```python
from build123d import *

# Parameters (mm, degrees)
SKETCH1_R           = 12.5
SKETCH1_R_2         = 1.6
SKETCH1_R_3         = 1
BOSS_EXTRUDE1_DEPTH = 5
CUT_EXTRUDE1_DEPTH  = 6
CIRPATTERN1_COUNT   = 22


with BuildPart() as part:
    # Sketch1 → Boss-Extrude1 (new body)
    with BuildSketch(Plane.XY):
        Circle(SKETCH1_R)
        Circle(SKETCH1_R_2, mode=Mode.SUBTRACT)
        with Locations((2.5, -7.4)):
            Circle(SKETCH1_R_3, mode=Mode.SUBTRACT)
        with Locations((-2.5, -7.4)):
            Circle(SKETCH1_R_3, mode=Mode.SUBTRACT)
        with Locations((7.4, -2.5)):
            Circle(SKETCH1_R_3, mode=Mode.SUBTRACT)
        with Locations((-7.4, -2.694035424)):
            Circle(SKETCH1_R_3, mode=Mode.SUBTRACT)
        with Locations((-7.4, 2.5)):
            Circle(SKETCH1_R_3, mode=Mode.SUBTRACT)
        with Locations((-2.5, 7.4)):
            Circle(SKETCH1_R_3, mode=Mode.SUBTRACT)
        with Locations((2.5, 7.4)):
            Circle(SKETCH1_R_3, mode=Mode.SUBTRACT)
        with Locations((7.4, 2.5)):
            Circle(SKETCH1_R_3, mode=Mode.SUBTRACT)
    extrude(amount=BOSS_EXTRUDE1_DEPTH)

    # Sketch2 → Cut-Extrude1 (cut, through all)
    with BuildSketch(Plane.XY.offset(5)):
        Polygon((-9.204992805, 8.456837911), (-6.616673599, 6.940063806), (-5.995627184, 7.483135026), (-7.153657676, 10.250618608), (-7.456074993, 10.596457577), (-9.507410122, 8.80267688), align=None)
    cut_extrude1 = extrude(amount=-CUT_EXTRUDE1_DEPTH, mode=Mode.SUBTRACT)

    # CirPattern1: Cut-Extrude1 ×22 about axis
    cirpattern1_axis = Axis((0, 0, 0), (0, 0, 1))
    for i in range(1, CIRPATTERN1_COUNT):
        add(cut_extrude1.rotate(cirpattern1_axis, i * 360 / CIRPATTERN1_COUNT), mode=Mode.SUBTRACT)


solid = part.part
```
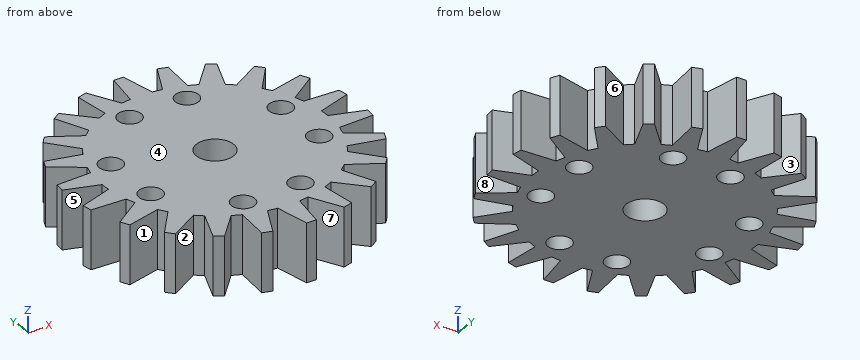
Here's how the part is built. I have some questions about the finished solid (model axes, mm). Face numbers are marked on the shaded views. A direction names the side the tool comes from. Give positions to 0.01 mm unless a question says otherwise; leave off trailing zeros. Write each loop counter-clockwise with the first axis right and the second up, starting at its lowest first coordinate (ties: lowest second). Pieces come first, ordered by that corner, then holes. Notation, with made-up numbers: M 85.25,40.25 L 120.25,40.25 A26 ccw 120.25,73.25 Z; hole C 15.25,-30 d2. An arc over 180 degrees is marked long. Put each result on its own line as item: value. Start each with the question number.
Item 1: Will this pin go through, and if not, where does the flat tip stop? pin 1 (2 mm diameter, centred on x = -7, z = 3, fed in from +Y).
Item 2: If we section it at D-D, the plane x = 2.5: Write out the boundary of the cut face in (y, z), then the cut area to 3 significant figures.
Item 3: I need wall thicknesses on L1, parallel to Y at x = 7.4, z = 1.85; L2, parallel to Y at x = 8.5, z = 0.35; L3, parallel to Y at x = 11.25, z = 2.45. Which ranges of each line are inside material? Lowest first, please. Write a range as from..to.
Item 4: If we section it at B-B, the plane x = 0: Write out the boundary of the cut face in (y, z), then the cut area to 3 significant figures.
Item 5: If we section it at C-C, the plane x = -2.75: Write out the boundary of the cut face in (y, z), then the cut area to 3 significant figures.
Item 6: Thinking about a two-plate mould opening in Y: for the marked faces 1, 2, 3 and 4, which applies, +Y half, -Y half, draft (parallel to the pull), parting line (faces both ways), or undercut?
Item 7: If we section it at A-A, the plane y = 0: Write out the boundary of the cut face in (x, z).
Item 8: On a 3-axis mill with a long thin cutter (end or side, diameter ignored), from which of +Z, -Z, +X, -X, +Y, -Y can I reach the whole of each face in a straight line? I mean the marked faces 5, 6, 7 and 8. Say none if no direction works.
Values:
1. pin 1: y = 10.71
2. outline: M -10.77,0 L -8.4,0 L -8.4,5 L -10.77,5 Z; M -6.4,0 L 6.4,0 L 6.4,5 L -6.4,5 Z; M 8.4,0 L 10.99,0 L 10.99,5 L 8.4,5 Z
2. area: 88.8 mm²
3. L1: -7.4..-3.5, -1.5..1.5, 3.5..7.51
3. L2: -8.04..-6.28, -4.84..4.93, 6.43..8.16
3. L3: -5.45..-4.54, -2.18..-0.92, 1.02..2.28, 4.67..5.45
4. outline: M -12.5,0 L -1.6,0 L -1.6,5 L -12.5,5 Z; M 1.6,0 L 12.5,0 L 12.5,5 L 1.6,5 Z
4. area: 109 mm²
5. outline: M -11.49,0 L -8.37,0 L -8.37,5 L -11.49,5 Z; M -6.43,0 L 6.43,0 L 6.43,5 L -6.43,5 Z; M 8.37,0 L 11.26,0 L 11.26,5 L 8.37,5 Z
5. area: 94.4 mm²
6. face 1: undercut
6. face 2: undercut
6. face 3: +Y half
6. face 4: draft
7. outline: M -9.58,0 L -1.6,0 L -1.6,5 L -9.58,5 Z; M 1.6,0 L 9.58,0 L 9.58,5 L 1.6,5 Z
8. face 5: +Z, -Z, -X
8. face 6: +Z, -Z
8. face 7: +Z, -Z, -Y
8. face 8: +Z, -Z, +X
